Autodesk Inventor part; units mm, degrees
ref_plane "YZ Plane" through (0, 0, 0) normal (1, 0, 0) x (0, 1, 0)
ref_plane "XZ Plane" through (0, 0, 0) normal (0, 1, 0) x (-1, 0, 0)
ref_plane "XY Plane" through (0, 0, 0) normal (0, 0, 1) x (1, 0, 0)
sketch "Esboço1" plane through (0, 0, 0) normal (0, 1, 0) x (-1, 0, 0)
  line L0 (0, 0) -> (72, 0)
  line L1 (72, 0) -> (72, -110)
  line L2 (72, -110) -> (0, -110)
  line L3 (0, -110) -> (0, 0)
  dimension "d0" = 72
  dimension "d1" = 110
extrude "Extrusão1" add sketch "Esboço1" along normal blind 6
sketch "Esboço2" plane through (0, 6, 0) normal (0, 1, 0) x (1, 0, 0)
  line L0 (0, 110) -> (-72, 110)
  line L1 (-72, 110) -> (-72, 0)
  line L2 (-72, 0) -> (0, 0)
  line L3 (0, 0) -> (0, 110)
  line L4 (-66, 104) -> (-6, 104)
  line L5 (-6, 104) -> (-6, 6)
  line L6 (-6, 6) -> (-66, 6)
  line L7 (-66, 6) -> (-66, 104)
  dimension "d4" = 6
extrude "Extrusão2" add sketch "Esboço2" along normal blind 44
sketch "Esboço3" plane through (-72, 0, 0) normal (0, 0, 1) x (1, 0, 0)
  circle A0 centre (23.5, 25) radius 8
  circle A1 centre (48.5, 25) radius 8
  line L0 (0, 50) -> (72, 50)
  line L1 (0, 0) -> (0, 50)
  line L2 (23.5, 25) -> (48.5, 25) construction
  point P0 (72, 0)
  point P1 (0, 25)
  point P2 (36, 25)
  point P3 (36, 50)
  dimension "d8" = 16
  dimension "d9" = 25
extrude "Extrusão3" cut sketch "Esboço3" against normal up to surface (6 mm away)
sketch "Esboço4" plane through (0, 0, 0) normal (1, 0, 0) x (0, 0, -1)
  line L0 (22.03, 11.6) -> (28.37, 11.6)
  arc A0 (28.37, 11.6) -> (29.67, 12.9) centre (28.37, 12.9) ccw
  line L1 (29.67, 12.9) -> (29.67, 13.46)
  arc A1 (29.67, 13.46) -> (28.37, 14.76) centre (28.37, 13.46) ccw
  line L2 (22.03, 14.76) -> (28.37, 14.76)
  arc A2 (22.03, 14.76) -> (20.73, 13.46) centre (22.03, 13.46) ccw
  line L3 (20.73, 12.9) -> (20.73, 13.46)
  arc A3 (20.73, 12.9) -> (22.03, 11.6) centre (22.03, 12.9) ccw
  arc A4 (28.37, 11.9) -> (29.37, 12.9) centre (28.37, 12.9) ccw
  line L4 (28.37, 11.9) -> (22.03, 11.9)
  arc A5 (21.03, 12.9) -> (22.03, 11.9) centre (22.03, 12.9) ccw
  line L5 (21.03, 13.46) -> (21.03, 12.9)
  arc A6 (22.03, 14.46) -> (21.03, 13.46) centre (22.03, 13.46) ccw
  line L6 (22.03, 14.46) -> (28.37, 14.46)
  arc A7 (29.37, 13.46) -> (28.37, 14.46) centre (28.37, 13.46) ccw
  line L7 (29.37, 12.9) -> (29.37, 13.46)
  line L8 (37.8445, 11.75) -> (39.84, 11.75)
  arc A8 (37.6268, 11.8436) -> (37.8445, 11.75) centre (37.8445, 12.05) ccw
  line L9 (36.9823, 12.5234) -> (37.6268, 11.8436)
  arc A9 (36.9, 12.7298) -> (36.9823, 12.5234) centre (37.2, 12.7298) ccw
  line L10 (36.9, 14.05) -> (36.9, 12.7298)
  arc A10 (37.2, 14.35) -> (36.9, 14.05) centre (37.2, 14.05) ccw
  line L11 (42.8, 14.35) -> (37.2, 14.35)
  arc A11 (43.1, 14.05) -> (42.8, 14.35) centre (42.8, 14.05) ccw
  line L12 (43.1, 12.7298) -> (43.1, 14.05)
  arc A12 (43.0177, 12.5234) -> (43.1, 12.7298) centre (42.8, 12.7298) ccw
  line L13 (42.3732, 11.8436) -> (43.0177, 12.5234)
  arc A13 (42.1555, 11.75) -> (42.3732, 11.8436) centre (42.1555, 12.05) ccw
  line L14 (40.16, 11.75) -> (42.1555, 11.75)
  line L15 (40.16, 11.6) -> (40.16, 11.75)
  line L16 (42.1555, 11.6) -> (40.16, 11.6)
  arc A14 (42.1555, 11.6) -> (42.4821, 11.7404) centre (42.1555, 12.05) ccw
  line L17 (43.1266, 12.4202) -> (42.4821, 11.7404)
  arc A15 (43.1266, 12.4202) -> (43.25, 12.7298) centre (42.8, 12.7298) ccw
  line L18 (43.25, 14.05) -> (43.25, 12.7298)
  arc A16 (43.25, 14.05) -> (42.8, 14.5) centre (42.8, 14.05) ccw
  line L19 (37.2, 14.5) -> (42.8, 14.5)
  arc A17 (37.2, 14.5) -> (36.75, 14.05) centre (37.2, 14.05) ccw
  line L20 (36.75, 12.7298) -> (36.75, 14.05)
  arc A18 (36.75, 12.7298) -> (36.8734, 12.4202) centre (37.2, 12.7298) ccw
  line L21 (37.5179, 11.7404) -> (36.8734, 12.4202)
  arc A19 (37.5179, 11.7404) -> (37.8445, 11.6) centre (37.8445, 12.05) ccw
  line L22 (39.84, 11.6) -> (37.8445, 11.6)
  line L23 (39.84, 11.75) -> (39.84, 11.6)
  line L24 (51.3445, 11.75) -> (53.34, 11.75)
  arc A20 (51.1268, 11.8436) -> (51.3445, 11.75) centre (51.3445, 12.05) ccw
  line L25 (50.4823, 12.5234) -> (51.1268, 11.8436)
  arc A21 (50.4, 12.7298) -> (50.4823, 12.5234) centre (50.7, 12.7298) ccw
  line L26 (50.4, 14.05) -> (50.4, 12.7298)
  arc A22 (50.7, 14.35) -> (50.4, 14.05) centre (50.7, 14.05) ccw
  line L27 (56.3, 14.35) -> (50.7, 14.35)
  arc A23 (56.6, 14.05) -> (56.3, 14.35) centre (56.3, 14.05) ccw
  line L28 (56.6, 12.7298) -> (56.6, 14.05)
  arc A24 (56.5177, 12.5234) -> (56.6, 12.7298) centre (56.3, 12.7298) ccw
  line L29 (55.8732, 11.8436) -> (56.5177, 12.5234)
  arc A25 (55.6555, 11.75) -> (55.8732, 11.8436) centre (55.6555, 12.05) ccw
  line L30 (53.66, 11.75) -> (55.6555, 11.75)
  line L31 (53.66, 11.6) -> (53.66, 11.75)
  line L32 (55.6555, 11.6) -> (53.66, 11.6)
  arc A26 (55.6555, 11.6) -> (55.9821, 11.7404) centre (55.6555, 12.05) ccw
  line L33 (56.6266, 12.4202) -> (55.9821, 11.7404)
  arc A27 (56.6266, 12.4202) -> (56.75, 12.7298) centre (56.3, 12.7298) ccw
  line L34 (56.75, 14.05) -> (56.75, 12.7298)
  arc A28 (56.75, 14.05) -> (56.3, 14.5) centre (56.3, 14.05) ccw
  line L35 (50.7, 14.5) -> (56.3, 14.5)
  arc A29 (50.7, 14.5) -> (50.25, 14.05) centre (50.7, 14.05) ccw
  line L36 (50.25, 12.7298) -> (50.25, 14.05)
  arc A30 (50.25, 12.7298) -> (50.3734, 12.4202) centre (50.7, 12.7298) ccw
  line L37 (51.0179, 11.7404) -> (50.3734, 12.4202)
  arc A31 (51.0179, 11.7404) -> (51.3445, 11.6) centre (51.3445, 12.05) ccw
  line L38 (53.34, 11.6) -> (51.3445, 11.6)
  line L39 (53.34, 11.75) -> (53.34, 11.6)
  line L40 (64.5, 17.6) -> (64.5, 11.6)
  line L41 (68, 11.6) -> (64.5, 11.6)
  arc A32 (68, 17.6) -> (68, 11.6) centre (68, 14.6) ccw
  line L42 (68, 17.6) -> (64.5, 17.6)
  line L43 (71.5, 17.6) -> (68, 17.6)
  arc A33 (68, 11.6) -> (68, 17.6) centre (68, 14.6) ccw
  line L44 (71.5, 11.6) -> (68, 11.6)
  line L45 (71.5, 11.6) -> (71.5, 17.6)
  circle A34 centre (68, 14.6) radius 4
  point P0 (0, 0)
  dimension "d12" = 1
extrude "Extrusão4" cut sketch "Esboço4" against normal up to next contours A34 L42 A32 L41 L40 | L40 A34 | A34 L43 L42 | A33 A32 | L43 A34 L45 L44 A33 | L41 L44 A34 | A34 L45
sketch "Esboço6" plane through (0, 50, 0) normal (0, 1, 0) x (1, 0, 0)
  line L0 (-72, 110) -> (-72, 0)
  line L1 (-72, 0) -> (0, 0)
  line L2 (0, 0) -> (0, 110)
  line L3 (0, 110) -> (-72, 110)
  line L4 (-66, 104) -> (-6, 104)
  line L5 (-6, 104) -> (-6, 6)
  line L6 (-6, 6) -> (-66, 6)
  line L7 (-66, 6) -> (-66, 104)
extrude "Extrusão5" add sketch "Esboço6" against normal blind 6 contours L4 L5 L6 L7
sketch "Esboço7" plane through (0, 0, 0) normal (1, 0, 0) x (0, 0, -1)
  line L0 (0, 0) -> (110, 0)
  line L1 (6, 6) -> (104, 6)
  line L2 (35, 0) -> (75, 0)
  line L3 (75, 0) -> (75, 6)
  line L4 (75, 6) -> (35, 6)
  line L5 (35, 6) -> (35, 0)
  point P0 (55, 6)
  point P1 (35, 6)
  point P2 (75, 0)
  dimension "d17" = 40
extrude "Extrusão6" add sketch "Esboço7" along normal blind 35
fillet "Arredondamento1" radius 10 4 edges at (0, 3, -35) (0, 3, -75) (35, 3, -75) (35, 3, -35)
ref_plane "Plano de trabalho1" through (-36, 0, -110) normal (1, 0, 0) x (0, 0, -1)
sketch "Esboço8" plane through (0, 6, -25) normal (0, 1, 0) x (1, 0, 0)
  circle A0 centre (17.5, 30) radius 5
  arc A1 (25, 10) -> (35, 20) centre (25, 20) ccw
  line L0 (35, 40) -> (35, 20)
  arc A2 (35, 40) -> (25, 50) centre (25, 40) ccw
  line L1 (10, 50) -> (25, 50)
  arc A3 (0, 60) -> (10, 50) centre (10, 60) ccw
  line L2 (0, 0) -> (0, 60)
  arc A4 (10, 10) -> (0, 0) centre (10, 0) ccw
  line L3 (10, 10) -> (25, 10)
  point P0 (0, -25)
  point P1 (35, 30)
  point P2 (17.5, 50)
  dimension "d21" = 10
extrude "Extrusão7" cut sketch "Esboço8" against normal blind 35 contours A0
mirror "Espelhar2" about plane through (-36, 0, -110) normal (1, 0, 0) of "Extrusão6", "Extrusão7"
fillet "Arredondamento2" radius 10 4 edges at (-72, 3, -35) (-107, 3, -35) (-107, 3, -75) (-72, 3, -75)
properties part number "Prototipo"
Build history of the part. All positions in model axes, mm. A direction names the side the tool comes from. Give positions to 0.01 mm unless a question says otherwise; leave off trailing zeros. Loops run counter-clockwise (first coordinate to the right, second up) from the corner with the lowest first, then second, coordinate; pieces in that order, holes last. Notation, with made-up numbers: (33, 86) - (73, 86) arc R34 cw to (73, 124) - close; hole circle Ø3 at (13, 9). An arc over 180 degrees is marked (long way). Use a Markdown table: item, result.
(1) Band-saw the part on C-C (y = 29). Give the cut face in (x, z), and give its area (3 significant figures).
Taken from the geometry:
| item | result |
|---|---|
| outline | (-72, -110) - (0, -110) - (0, 0) - (-16.57, 0) - (-16.57, -6) - (-6, -6) - (-6, -104) - (-66, -104) - (-66, -6) - (-55.43, -6) - (-55.43, 0) - (-72, 0) - close; (-41.57, -6) - (-30.43, -6) - (-30.43, 0) - (-41.57, 0) - close |
| area | 1,870 mm2 |
(2) Pull direction Z, two halves, no side cores. Call faces 5 (the face through (-35, 0, -54)), 6 (the face through (-75.01, 3.04, -77.85)), 7 (the face through (-2.958, 13.068, -71.695)): +Z half, -Z half, draft (parallel to the pull), parting line (faces both ways), or undercut.
Taken from the geometry:
| item | result |
|---|---|
| face 5 | draft |
| face 6 | -Z half |
| face 7 | undercut |
(3) Band-saw the part on D-D (x = -33). Give the cut face in (y, z), and give its area (3 significant figures).
Taken from the geometry:
| item | result |
|---|---|
| outline | (0, -110) - (50, -110) - (50, 0) - (0, 0) - close; hole (6, -104) - (44, -104) - (44, -6) - (6, -6) - close |
| area | 1,780 mm2 |
(4) Which spindle directions (+Z, -Z, +X, -X, +Y, -Y) get a long thin tool onto all of the face, cutting with end or side? Do faces 1 (the face through (-89, 3, -75)), 2 (the face through (-24.541, 32.932, -2.958)), 3 (the face through (-89, 6, -49)), 4 (the face through (-6, 25, -56)). Say none if no direction does.
Taken from the geometry:
| item | result |
|---|---|
| face 1 | -Z, -X, +Y, -Y |
| face 2 | +Z |
| face 3 | +Z, -Z, -X, +Y |
| face 4 | none |
(5) Band-saw the part on B-B (x = -89.5). Give the cut face in (y, z).
Taken from the geometry:
| item | result |
|---|---|
| outline | (0, -75) - (6, -75) - (6, -60) - (0, -60) - close; (0, -50) - (6, -50) - (6, -35) - (0, -35) - close |
(6) Band-saw the part on A-A (z = -58). Give the cut face in (x, y), and give its area (3 significant figures).
Taken from the geometry:
| item | result |
|---|---|
| outline | (-107, 0) - (-93.5, 0) - (-93.5, 6) - (-107, 6) - close; (-85.5, 0) - (13.5, 0) - (13.5, 6) - (0, 6) - (0, 50) - (-72, 50) - (-72, 6) - (-85.5, 6) - close; (21.5, 0) - (35, 0) - (35, 6) - (21.5, 6) - close; hole (-66, 6) - (-6, 6) - (-6, 44) - (-66, 44) - close |
| area | 1,640 mm2 |
(7) Drop flat-ended pins along their axis: pin 1 Ø6.5 at (x, y) = (18.5, 2) entering from +Z; pin 2 Ø8 at (y, z) = (7.5, -36.5) entering from +X; pin 3 Ø6 at (x, z) = (17.5, -55) entering from +Y; pin 4 Ø3 at (x, y) = (14, 4.5) entering from -Z. Give the stop position or say it passes through.
Taken from the geometry:
| item | result |
|---|---|
| pin 1 | z = -35 |
| pin 2 | x = 33.78 |
| pin 3 | through |
| pin 4 | z = -75 |
(8) Wall check: line 1 along X through (y, z) = (4.2, -55); line 2 along Y through (x, z) = (-53, -30.5); line 3 along X through (y, z) = (21, -72.5). Give the ranges that are in metal, low to high.
Taken from the geometry:
| item | result |
|---|---|
| line 1 | -107 to -94.5, -84.5 to 12.5, 22.5 to 35 |
| line 2 | 0 to 6, 44 to 50 |
| line 3 | -72 to -66, -6 to 0 |
